```python
from build123d import *

# Parameters (mm, degrees)
F1_DEPTH = 2
F2_DEPTH = 5
F5_DEPTH = 18


# Not quite as in the source:
# - ends of sketch curves that miss each other by under 0.0002 mm in the source are joined


with BuildPart() as f1:
    # F0 (on Front) → F1 (new body)
    with BuildSketch(Plane.XZ):
        Polygon((13.9564371829, -4.1763302545), (13.6505568212, -1.5672102939), (13.8570021684, 0.6546701968), (14.4386421574, 2.572777133), (15.2749946567, 4.1916956816), (16.2455787436, 5.5160118155), (17.2299147044, 6.5503102987), (18.1075224224, 7.29917791), (18.7579217808, 7.7671990103), (19.0606326631, 7.9589595725), (17.8894090385, 9.4061765559), (16.6182390109, 10.5424416074), (15.3009021796, 11.4051715106), (13.991178144, 12.0317814369), (12.7428465032, 12.45968817), (11.6096864535, 12.7263080903), (10.6454779973, 12.8690567726), (9.9040003307, 12.9253510002), (8.4536993007, 12.9401075165), (7.0393171578, 12.7333035124), (5.6789414949, 12.3726223866), (4.3906586959, 11.9257463288), (4.0349177671, 11.7875631309), (3.1925567568, 11.4603583345), (2.1027220613, 11.0441405935), (1.1392422025, 10.7447756984), (1.0630562956, 10.7340944764), (0.3202043703, 10.6299470477), (-0.4697068924, 10.7259466125), (-1.3499739104, 10.9785104051), (-2.3101170508, 11.3344870803), (-3.3396570834, 11.740725293), (-4.428114778, 12.144073295), (-5.5650109045, 12.4913797411), (-6.7398666357, 12.7294928833), (-7.9422027416, 12.8052613763), (-9.5179845331, 12.6738502829), (-11.0461403111, 12.3335924529), (-12.5103628719, 11.7956320422), (-13.8943458175, 11.0711148186), (-15.1817823473, 10.171185744), (-16.3563656605, 9.1069897803), (-17.4017889563, 7.8896718894), (-18.3017458369, 6.530377436), (-19.6083064378, 3.5020943147), (-20.2715944756, 0.231420362), (-20.3699313552, -3.1782734497), (-19.9816400935, -6.6236177604), (-19.1850429015, -10.0012415978), (-18.0584619901, -13.2077743927), (-16.6802199733, -16.139845979), (-15.1286390619, -18.6940861905), (-14.3199712507, -19.8437521157), (-13.468975877, -20.9834397215), (-12.5711806097, -22.0670519206), (-11.6221131177, -23.0484932379), (-10.617301876, -23.881667795), (-9.5522737476, -24.5204789077), (-8.4225572075, -24.9188306978), (-6.2785486616, -24.924760094), (-6.1172446521, -24.9066919741), (-5.1420524281, -24.6576772732), (-4.2440729965, -24.3272277028), (-3.3692761011, -23.9589889904), (-2.4636318887, -23.5966060577), (-1.4731105063, -23.2837238261), (-0.3436821007, -23.0639884263), (0.9786835843, -22.9810443767), (2.2966708338, -23.0689926979), (3.415326636, -23.3003344778), (4.3935835633, -23.6263149411), (5.2903729793, -23.9981789094), (6.1646270535, -24.3671716073), (7.0752771494, -24.6845382594), (8.0812554366, -24.9015236875), (9.211135995, -24.9675978327), (9.2543495324, -24.9677173425), (10.4646266505, -24.8118393056), (11.5846824237, -24.4101431404), (12.6153226062, -23.7990147009), (13.5702096091, -23.0131824556), (14.4630054406, -22.087375679), (15.3073721089, -21.0563232426), (16.1169720251, -19.9547548237), (16.9054676003, -18.817399697), (17.7450979821, -17.5059903767), (18.4573257656, -16.2416880249), (19.0477701778, -15.0611340813), (19.522050849, -14.0009703886), (19.8857874094, -13.0978387898), (20.1446002953, -12.3883807244), (20.3041087338, -11.9092380354), (20.3699323552, -11.6970525654), (20.0632597243, -11.5632690975), (19.2992902384, -11.1660557409), (18.2304933913, -10.4753497913), (17.0093394832, -9.461087335), (15.7882988139, -8.0932056676), (14.7198412805, -6.3416408756), align=None)
        Polygon((3.1925567568, 11.4603583345), (4.0349177671, 11.7875631309), (4.0349177671, 14.3890940084), (3.0470887296, 13.9600045134), (2.0233786856, 13.6566557055), (0.9776241359, 13.4953402808), (1.0630562956, 10.7340944764), (1.1392422025, 10.7447756984), (2.1027220613, 11.0441405935), align=None)
        Polygon((3.0470887296, 13.9600045134), (4.0349177671, 14.3890940084), (4.9730284914, 14.9276318971), (5.8475844015, 15.5593258862), (6.6447481909, 16.2678824734), (7.3506829556, 17.0370097684), (7.9776442852, 17.8678175927), (8.5401819643, 18.7665723681), (9.0274431955, 19.7233570289), (9.4285759872, 20.7282545094), (9.7327275419, 21.7713473411), (9.9290458681, 22.8427184583), (10.0066785712, 23.9324507955), (9.9547732566, 25.030626884), (8.9884152767, 24.9252998211), (7.9933494289, 24.6925222045), (6.9902835166, 24.3433068169), (5.9999257462, 23.888667247), (5.0429839212, 23.3396154714), (4.1401666508, 22.7071646759), (3.3121821416, 22.0023272402), (2.5797377939, 21.2361167529), (1.9848069462, 20.4835481245), (1.4275088821, 19.6401188001), (0.9265880606, 18.7204873704), (0.5007873288, 17.7393128294), (0.1688511456, 16.7112529619), (-0.0504776421, 15.6509671648), (-0.1384553812, 14.5731136257), (-0.0763380157, 13.4923513387), (0.9776241359, 13.4953402808), (2.0233786856, 13.6566557055), align=None)
    extrude(amount=F1_DEPTH)

    # F0 (on Front) → F2 (join)
    with BuildSketch(Plane.XZ):
        Polygon((13.9564371829, -4.1763302545), (13.6505568212, -1.5672102939), (13.8570021684, 0.6546701968), (14.4386421574, 2.572777133), (15.2749946567, 4.1916956816), (16.2455787436, 5.5160118155), (17.2299147044, 6.5503102987), (18.1075224224, 7.29917791), (18.7579217808, 7.7671990103), (19.0606326631, 7.9589595725), (17.8894090385, 9.4061765559), (16.6182390109, 10.5424416074), (15.3009021796, 11.4051715106), (13.991178144, 12.0317814369), (12.7428465032, 12.45968817), (11.6096864535, 12.7263080903), (10.6454779973, 12.8690567726), (9.9040003307, 12.9253510002), (8.4536993007, 12.9401075165), (7.0393171578, 12.7333035124), (5.6789414949, 12.3726223866), (4.3906586959, 11.9257463288), (4.0349177671, 11.7875631309), (3.1925567568, 11.4603583345), (2.1027220613, 11.0441405935), (1.1392422025, 10.7447756984), (1.0630562956, 10.7340944764), (0.3202043703, 10.6299470477), (-0.4697068924, 10.7259466125), (-1.3499739104, 10.9785104051), (-2.3101170508, 11.3344870803), (-3.3396570834, 11.740725293), (-4.428114778, 12.144073295), (-5.5650109045, 12.4913797411), (-6.7398666357, 12.7294928833), (-7.9422027416, 12.8052613763), (-9.5179845331, 12.6738502829), (-11.0461403111, 12.3335924529), (-12.5103628719, 11.7956320422), (-13.8943458175, 11.0711148186), (-15.1817823473, 10.171185744), (-16.3563656605, 9.1069897803), (-17.4017889563, 7.8896718894), (-18.3017458369, 6.530377436), (-19.6083064378, 3.5020943147), (-20.2715944756, 0.231420362), (-20.3699313552, -3.1782734497), (-19.9816400935, -6.6236177604), (-19.1850429015, -10.0012415978), (-18.0584619901, -13.2077743927), (-16.6802199733, -16.139845979), (-15.1286390619, -18.6940861905), (-14.3199712507, -19.8437521157), (-13.468975877, -20.9834397215), (-12.5711806097, -22.0670519206), (-11.6221131177, -23.0484932379), (-10.617301876, -23.881667795), (-9.5522737476, -24.5204789077), (-8.4225572075, -24.9188306978), (-6.2785486616, -24.924760094), (-6.1172446521, -24.9066919741), (-5.1420524281, -24.6576772732), (-4.2440729965, -24.3272277028), (-3.3692761011, -23.9589889904), (-2.4636318887, -23.5966060577), (-1.4731105063, -23.2837238261), (-0.3436821007, -23.0639884263), (0.9786835843, -22.9810443767), (2.2966708338, -23.0689926979), (3.415326636, -23.3003344778), (4.3935835633, -23.6263149411), (5.2903729793, -23.9981789094), (6.1646270535, -24.3671716073), (7.0752771494, -24.6845382594), (8.0812554366, -24.9015236875), (9.211135995, -24.9675978327), (9.2543495324, -24.9677173425), (10.4646266505, -24.8118393056), (11.5846824237, -24.4101431404), (12.6153226062, -23.7990147009), (13.5702096091, -23.0131824556), (14.4630054406, -22.087375679), (15.3073721089, -21.0563232426), (16.1169720251, -19.9547548237), (16.9054676003, -18.817399697), (17.7450979821, -17.5059903767), (18.4573257656, -16.2416880249), (19.0477701778, -15.0611340813), (19.522050849, -14.0009703886), (19.8857874094, -13.0978387898), (20.1446002953, -12.3883807244), (20.3041087338, -11.9092380354), (20.3699323552, -11.6970525654), (20.0632597243, -11.5632690975), (19.2992902384, -11.1660557409), (18.2304933913, -10.4753497913), (17.0093394832, -9.461087335), (15.7882988139, -8.0932056676), (14.7198412805, -6.3416408756), align=None)
        Polygon((3.0470887296, 13.9600045134), (4.0349177671, 14.3890940084), (4.9730284914, 14.9276318971), (5.8475844015, 15.5593258862), (6.6447481909, 16.2678824734), (7.3506829556, 17.0370097684), (7.9776442852, 17.8678175927), (8.5401819643, 18.7665723681), (9.0274431955, 19.7233570289), (9.4285759872, 20.7282545094), (9.7327275419, 21.7713473411), (9.9290458681, 22.8427184583), (10.0066785712, 23.9324507955), (9.9547732566, 25.030626884), (8.9884152767, 24.9252998211), (7.9933494289, 24.6925222045), (6.9902835166, 24.3433068169), (5.9999257462, 23.888667247), (5.0429839212, 23.3396154714), (4.1401666508, 22.7071646759), (3.3121821416, 22.0023272402), (2.5797377939, 21.2361167529), (1.9848069462, 20.4835481245), (1.4275088821, 19.6401188001), (0.9265880606, 18.7204873704), (0.5007873288, 17.7393128294), (0.1688511456, 16.7112529619), (-0.0504776421, 15.6509671648), (-0.1384553812, 14.5731136257), (-0.0763380157, 13.4923513387), (0.9776241359, 13.4953402808), (2.0233786856, 13.6566557055), align=None)
    extrude(amount=F2_DEPTH)

    # F4 (on line) → F5 (join)
    with BuildSketch(Plane(origin=(9.921820884, 0, -0.0274394463), x_dir=(0, 1, 0), z_dir=(0.9999961758, 0, -0.002765555))):
        Polygon((0, -24.9420284495), (-2.5, -24.9420284495), (-2.5, -34.9420284495), (5, -34.9420284495), (5, -32.4420284495), (2.5, -32.4420284495), align=None)
        Polygon((-2.5, -24.9420284495), (-5, -24.9420284495), (-7.5, -32.4420284495), (-10, -32.4420284495), (-10, -34.9420284495), (-2.5, -34.9420284495), align=None)
        Polygon((-5, -23.9420284495), (-5, -24.9420284495), (-2.5, -24.9420284495), (0, -24.9420284495), (0, -23.9420284495), align=None)
    extrude(amount=-F5_DEPTH)


solid = f1.part
```
For this review, take the finished solid that the model builds, in its own axes (mm). A direction names the side the tool comes from. Coordinates: 2 decimals unless noted, no trailing zeros. Loops run counter-clockwise (first coordinate to the right, second up) from the corner with the lowest first, then second, coordinate; pieces in that order, holes last. Notation, with made-up numbers: (35.5, 52.5) - (84.5, 52.5) arc R14 cw to (84.5, 62.5) - close; hole circle Ø3 at (88.25, 61). An arc over 180 degrees is marked (long way). Use one line per item in the form item = value. Start each with the question number.
1) Take a section at C-C (z = -27). State the section outline as (x, y) points.
2) For faces 4 (the face through (14.34, -2.46, -5.27)), 5 (the face through (0, -5, -6)), 6 (the face through (-7.333, -2.465, 12.767)), 7 (the face through (-0.916, -2.465, -23.175)), 8 (the face through (-19.935, -2.465, 1.89)), list the 3-axis set-ups (+Z, -Z, +X, -X, +Y, -Y) from which the entire face can be reached by the end or side of a thin tool; tool diameter is ignored.
3) To check wall thickness, follow probe 1 along Y at (x, z) = (6.5, 17); probe 2 along Z at (x, y) = (-5, -8); probe 3 along Z at (x, y) = (5, 3.5). State the ranges of each line that lie inside material, in increasing order. Write a range as from..to.
4) Take a section at A-A (y = -3.75). State how many separate pieces and enclosed holes the cut face has, plus the area to 3 significant figures.
5) For pin 1 (3 mm diameter, centred on x = -0.5, z = -16.5, fed in from -Y); pin 2 (2 mm diameter, centred on y = -1, z = 12.5, fed in from +X); pin 3 (2 mm diameter, centred on x = 7.5, z = -1.5, fed in from +Y), all flat-tipped, find the tip position at first contact; note any pin that passes through.
6) Draft analysis for pull direction Z (two halves, no side actions). For faces 1 (the face through (17.628, -2.465, -9.975)), 2 (the face through (18.483, -2.465, 8.672)), 3 (the face through (17.3, -2.5, -18.2)), state which applies: released by +Z, released by -Z, zero draft, split by the parting line, or undercut.
7) Take a section at B-B (y = 3.25). State the section outline as (x, z) points, plus the area to 3 significant figures.
From the geometry:
q1.outline = (-8.15, -5.69) - (9.85, -5.68) - (9.85, 0.68) - (-8.15, 0.69) - close
q2.face_4 = +X, +Y, -Y
q2.face_5 = +Z, +X, -X, -Y
q2.face_6 = +Z, +Y, -Y
q2.face_7 = +Y, -Y
q2.face_8 = +Z, -X, +Y, -Y
q3.probe_1 = -5..0
q3.probe_2 = -34.93..-32.43
q3.probe_3 = -34.96..-32.46
q4.separate_pieces = 2
q4.enclosed_holes = 1
q4.area = 1,480 mm2
q5.pin_1 = -5
q5.pin_2 = 15.1
q5.pin_3 = 0
q6.face_1 = undercut
q6.face_2 = released by +Z
q6.face_3 = released by -Z
q7.outline = (-8.17, -34.92) - (9.83, -34.97) - (9.83, -32.47) - (-8.17, -32.42) - close
q7.area = 45.0 mm2
